from build123d import *

# Parameters (mm, degrees)
F0_W      = 1400
F0_H      = 200
F0_W_2    = 40
F0_H_2    = 120
F1_DEPTH  = 40
F2_W      = 40
F2_H      = 40
F3_DEPTH  = 400
F4_W      = 40
F4_H      = 40
F5_DEPTH  = 200
F7_W      = 40
F7_H      = 40
F6_W      = 40
F6_H      = 40
F8_DEPTH  = 180
F9_W      = 40
F9_H      = 40
F10_DEPTH = 1320


# Not quite as in the source:
# - a feature names something its author has since deleted; it is built from what else it names


with BuildPart() as f1:
    # F0 (on Top) → F1 (new body)
    with BuildSketch(Plane.XY):
        Rectangle(F0_W, F0_H)
        Polygon((20, 60), (660, 60), (660, -60), (20, -60), (-20, -60), (-660, -60), (-660, 60), (-20, 60), align=None, mode=Mode.SUBTRACT)
        Rectangle(F0_W_2, F0_H_2)
    extrude(amount=F1_DEPTH)

    # F2 (on face) → F3 (join)
    with BuildSketch(Plane(origin=(0, 0, 0), x_dir=(1, 0, 0), z_dir=(0, 0, -1))):
        with Locations((-680, 80)):
            Rectangle(F2_W, F2_H)
        with Locations((-680, -80)):
            Rectangle(F2_W, F2_H)
        with Locations((680, 80)):
            Rectangle(F2_W, F2_H)
        with Locations((680, -80)):
            Rectangle(F2_W, F2_H)
        with Locations((0, 80)):
            Rectangle(F2_W, F2_H)
    extrude(amount=F3_DEPTH)

    # F4 (on face) → F5 (join)
    with BuildSketch(Plane(origin=(0, 100, 0), x_dir=(-1, 0, 0), z_dir=(0, 1, 0))):
        with Locations((-680, -200)):
            Rectangle(F4_W, F4_H)
        with Locations((680, -200)):
            Rectangle(F4_W, F4_H)
    extrude(amount=F5_DEPTH)

    # F7 (on face) + F6 (on face) → F8 (join)
    with BuildSketch(Plane(origin=(0, 0, -220), x_dir=(1, 0, 0), z_dir=(0, 0, -1))):
        with Locations((680, -280)):
            Rectangle(F7_W, F7_H)
    with BuildSketch(Plane(origin=(0, 0, -220), x_dir=(1, 0, 0), z_dir=(0, 0, -1))):
        with Locations((-680, -280)):
            Rectangle(F6_W, F6_H)
    extrude(amount=F8_DEPTH)

    # F9 (on face) → F10 (join, through all)
    with BuildSketch(Plane(origin=(660, 0, 0), x_dir=(0, -1, 0), z_dir=(-1, 0, 0))):
        with Locations((-280, -200)):
            Rectangle(F9_W, F9_H)
    extrude(amount=F10_DEPTH)


solid = f1.part
Design review of the part built by this model. Coordinates are the model's own, in mm. A direction names the side the tool comes from. Give positions to 0.01 mm unless a question says otherwise; leave off trailing zeros. Loops run counter-clockwise (first coordinate to the right, second up) from the corner with the lowest first, then second, coordinate; pieces in that order, holes last. Notation, with made-up numbers: (61.25, 28.5) - (83.25, 28.5) arc R26 ccw to (83.25, 46.5) - close; hole circle Ø9 at (23.25, 5). An arc over 180 degrees is marked (long way). Use CSV: the item, a comma, the result in double quotes. Start each with the question number.
1. Add section B-B (y = 0.5). State the section outline as (x, z) points.
2. Add section C-C (x = 485.5). State the section outline as (y, z) points, plus the area to 3 significant figures.
3. Wall thickness on L1, parallel to Y at x = -571, z = 12.5; L2, parallel to X at y = 277.5, z = -273.5; L3, parallel to Z at x = -159.5, y = 63: over which ranges is each line inside the solid? List them lowest first.
4. Machinability: for faces 1 (the flat face through (680, 179, -220)), 2 (the flat face through (20, -1, 20)), 3 (the flat face through (-3, 68, 0)), 4 (the flat face through (159, 267, -180)), 5 (the flat face through (-680, -80, -400)), which of the approach directions +Z, -Z, +X, -X, +Y, -Y give a long, thin tool a straight path to every point of the face, cutting with its end or side? Answer none if there is none.
5. Insertion check: P1, Ø12, axis at x = 201, y = 90.5, coming from the -Z side; P2, Ø20, axis at x = -277.5, z = 26, coming from the +Y side. Each pin has a flat end and moves straight along its axis. Give the tip position at first contact, or say it passes through.
6. Draft analysis for pull direction X (two halves, no side actions). For faces 6 (the flat face through (-680, -60, -197)), 7 (the flat face through (344, -60, 20)), state which applies: released by +X, released by -X, zero draft, split by the parting line, or undercut.
7. Add section A-A (z = -19). State the section outline as (x, y) points.
8. Add section D-D (z = -340.5). State the section outline as (x, y) points, plus the area to 3 significant figures.
Results found:
1,outline,"(-700, 0) - (-660, 0) - (-660, 40) - (-700, 40) - close; (-20, 0) - (20, 0) - (20, 40) - (-20, 40) - close; (660, 0) - (700, 0) - (700, 40) - (660, 40) - close"
2,outline,"(-100, 0) - (-60, 0) - (-60, 40) - (-100, 40) - close; (60, 0) - (100, 0) - (100, 40) - (60, 40) - close; (260, -220) - (300, -220) - (300, -180) - (260, -180) - close"
2,area,"4,800 mm²"
3,L1,"y = -100 to -60, 60 to 100"
3,L2,"x = -700 to -660, 660 to 700"
3,L3,"z = 0 to 40"
4,face 1,"-Z, +X, -X"
4,face 2,"+Z, -Z"
4,face 3,"-Z, +Y"
4,face 4,"+Z, +X, -X, +Y"
4,face 5,"-Z, +X, -X, +Y, -Y"
5,P1,"stops at z = 0"
5,P2,"stops at y = 100"
6,face 6,"zero draft"
6,face 7,"undercut"
7,outline,"(-700, -100) - (-660, -100) - (-660, -60) - (-700, -60) - close; (-700, 60) - (-660, 60) - (-660, 100) - (-700, 100) - close; (-20, -100) - (20, -100) - (20, -60) - (-20, -60) - close; (660, -100) - (700, -100) - (700, -60) - (660, -60) - close; (660, 60) - (700, 60) - (700, 100) - (660, 100) - close"
8,outline,"(-700, -100) - (-660, -100) - (-660, -60) - (-700, -60) - close; (-700, 60) - (-660, 60) - (-660, 100) - (-700, 100) - close; (-700, 260) - (-660, 260) - (-660, 300) - (-700, 300) - close; (-20, -100) - (20, -100) - (20, -60) - (-20, -60) - close; (660, -100) - (700, -100) - (700, -60) - (660, -60) - close; (660, 60) - (700, 60) - (700, 100) - (660, 100) - close; (660, 260) - (700, 260) - (700, 300) - (660, 300) - close"
8,area,"11,200 mm²"
